from build123d import *

# Parameters (mm, degrees)
SKETCH_4_W               = 60
SKETCH_4_H               = 35
SKETCH_4_R               = 5
EXTRUDE_1_DEPTH          = 10
FILLET_1_R               = 10
FILLET_2_R               = 10
EXTRUDE_2_DEPTH          = 8
SKETCH_6_R               = 15
EXTRUDE_3_DEPTH          = 30
SKETCH_8_R               = 10
CUT_EXTRUDE_1_DEPTH      = 74.484692283
EXTRUDE_4_REACH          = 76.33
EXTRUDE_4_END_RADIUS     = 15
SKETCH_9_R               = 7.5
CUT_EXTRUDE_2_REACH      = 76.33
CUT_EXTRUDE_2_END_RADIUS = 10
SKETCH_10_R              = 5
RIB_START                = -2.5
RIB_1_DEPTH              = 5


# Read off the part's stored shape, not the designer's step: 筋1
with BuildPart() as part:
    # 草图4 → 凸台-拉伸1 (new body)
    with BuildSketch(Plane(origin=(0, 0, 0), x_dir=(1, 0, 0), z_dir=(0, 1, 0))):
        with Locations((0, 2.5)):
            Rectangle(SKETCH_4_W, SKETCH_4_H)
        with Locations(Location((-20, -5, 0), (0, 0, 270))):
            Circle(SKETCH_4_R, mode=Mode.SUBTRACT)
        with Locations(Location((20, -5, 0), (0, 0, 90))):
            Circle(SKETCH_4_R, mode=Mode.SUBTRACT)
    extrude(amount=EXTRUDE_1_DEPTH)

    # 圆角1
    fillet_1_edges = [part.edges().sort_by_distance(p)[0] for p in [
        (-30, 5, 15),
    ]]
    fillet(fillet_1_edges, radius=FILLET_1_R)

    # 圆角2
    fillet_2_edges = [part.edges().sort_by_distance(p)[0] for p in [
        (30, 5, 15),
    ]]
    fillet(fillet_2_edges, radius=FILLET_2_R)

    # 草图5 → 凸台-拉伸2 (add)
    with BuildSketch(Plane(origin=(0, 0, -20), x_dir=(-1, 0, 0), z_dir=(0, 0, -1))):
        with BuildLine():
            Line((-30, 10), (-13.945515037, 50.524727174))
            ThreePointArc((-13.945515037, 50.524727174), (0, 60), (13.945515037, 50.524727174))
            Line((13.945515037, 50.524727174), (30, 10))
            Line((30, 10), (-30, 10))
        make_face()
    extrude(amount=-EXTRUDE_2_DEPTH)

    # 草图6 → 凸台-拉伸3 (add)
    with BuildSketch(Plane(origin=(0, 0, -20), x_dir=(-1, 0, 0), z_dir=(0, 0, -1))):
        with Locations((0, 45)):
            Circle(SKETCH_6_R)
    extrude(amount=-EXTRUDE_3_DEPTH)

    # 草图8 → 切除-拉伸1 (cut, through all)
    with BuildSketch(Plane.XY.offset(10)):
        with Locations((0, 45)):
            Circle(SKETCH_8_R)
    extrude(amount=-CUT_EXTRUDE_1_DEPTH, mode=Mode.SUBTRACT)

    # 凸台-拉伸4: up to this cylinder (the profile starts outside it)
    extrude_4_end = Plane(origin=(0, 45, 0), z_dir=(0, 0, -1)) * Cylinder(EXTRUDE_4_END_RADIUS, 183.66, mode=Mode.PRIVATE)
    # 草图9 → 凸台-拉伸4 (add, up to the surface)
    with BuildSketch(Plane(origin=(0, 65, 0), x_dir=(1, 0, 0), z_dir=(0, 1, 0)), mode=Mode.PRIVATE) as extrude_4_sk1:
        with Locations(Location((0, 0, 0), (0, 0, 270))):
            Circle(SKETCH_9_R)
    extrude_4_tool1 = extrude(extrude_4_sk1.sketch, amount=-EXTRUDE_4_REACH, mode=Mode.PRIVATE) - extrude_4_end
    add(extrude_4_tool1.solids().sort_by_distance((0, 65, 0))[0])

    # 切除-拉伸2: up to this cylinder (the profile starts outside it)
    cut_extrude_2_end = Plane(origin=(0, 45, 0), z_dir=(0, 0, 1)) * Cylinder(CUT_EXTRUDE_2_END_RADIUS, 173.66, mode=Mode.PRIVATE)
    # 草图10 → 切除-拉伸2 (cut, up to the surface)
    with BuildSketch(Plane(origin=(0, 65, 0), x_dir=(1, 0, 0), z_dir=(0, 1, 0)), mode=Mode.PRIVATE) as cut_extrude_2_sk1:
        with Locations(Location((0, 0, 0), (0, 0, 270))):
            Circle(SKETCH_10_R)
    cut_extrude_2_tool1 = extrude(cut_extrude_2_sk1.sketch, amount=-CUT_EXTRUDE_2_REACH, mode=Mode.PRIVATE) - cut_extrude_2_end
    add(cut_extrude_2_tool1.solids().sort_by_distance((0, 65, 0))[0], mode=Mode.SUBTRACT)

    # 筋1 outline → 筋1 (add)
    with BuildSketch(Plane(origin=(0, 0, 0), x_dir=(0, 0, -1), z_dir=(1, 0, 0)).offset(RIB_START)):
        Polygon((-5, 32), (-5, 20), (-15, 10), (12, 10), (12, 32), align=None)
    extrude(amount=RIB_1_DEPTH)


solid = part.part
Build history of the part. All positions in model axes, mm. A direction names the side the tool comes from. Round coordinates to 2 decimals unless told otherwise and drop trailing zeros. Loops run counter-clockwise (first coordinate to the right, second up) from the corner with the lowest first, then second, coordinate; pieces in that order, holes last. Notation, with made-up numbers: (-33, 46) -> (-11, 46) arc R15 cw to (-11, 51) -> close; hole circle Ø7 at (-40, 40). An arc over 180 degrees is marked (long way). One line per item, written item: value. Start each with the question number.
Q1. Cut at B-B on y = 47. List the corners of the cut face in (x, z).
Q2. Drop flat-ended pins along their axis: pin 1 Ø3 at (y, z) = (49.5, -2.5) entering from +X; pin 2 Ø8 at (x, z) = (0, 0) entering from +Y; pin 3 Ø5 at (x, y) = (13, 34.5) entering from +Z. Give the stop position or say it passes through.
Q3. Cut at A-A on x = 0. List the corners of the cut face in (y, z).
Q4. Two-plate mould, pull along X, no slides. Class faces 5 (the face through (-5, 65, 2)), 6 (the face through (-21.86, 30.55, -16.06)), 7 (the face through (24.88, 4.93, 6.08)): released by +X, released by -X, zero draft, split by the parting line, or undercut.
Q5. Cut at C-C on z = 2. List the corners of the cut face in (x, y).
Q6. Cut at D-D on x = -22. List the corners of the cut face in (y, z), plus the area to 3 significant figures.
Q7. Probe line 1 along Z through (x, y) = (20, 5); line 2 along Z through (x, y) = (0, 62.25). List the from-to ranges inside material, lowest first.
Q8. 3-axis set-ups, long thin cutter, end or side, ignore diameter. For faces 1 (the face through (1.5, 59.41, 4.77)), 2 (the face through (2.5, 20, -1)), 3 (the face through (-16, 10, 1)), 4 (the face through (0, 15, 10)): which of +Z, -Z, +X, -X, +Y, -Y reach the whole face in a straight line?
Computed:
1. outline: (-15.34, -20) -> (-9.8, -20) -> (-9.8, 10) -> (-14.87, 10) -> (-14.87, -12) -> (-15.34, -12) -> close; (9.8, -20) -> (15.34, -20) -> (15.34, -12) -> (14.87, -12) -> (14.87, 10) -> (9.8, 10) -> close
2. pin 1: x = 14.7
2. pin 2: y = 35.83
2. pin 3: z = 10
3. outline: (0, -20) -> (35, -20) -> (35, 10) -> (30, 10) -> (30, 5) -> (20, 5) -> (10, 15) -> (0, 15) -> close; (55, -20) -> (60, -20) -> (60, -7.5) -> (65, -7.5) -> (65, -5) -> (55, -5) -> close; (55, 5) -> (65, 5) -> (65, 7.5) -> (60, 7.5) -> (60, 10) -> (55, 10) -> close
4. face 5: zero draft
4. face 6: released by -X
4. face 7: undercut
5. outline: (-30, 0) -> (-24, 0) -> (-24, 10) -> (-30, 10) -> close; (-16, 0) -> (16, 0) -> (16, 10) -> (2.5, 10) -> (2.5, 30.21) arc R15 ccw to (7.23, 58.14) -> (7.23, 65) -> (4.58, 65) -> (4.58, 53.89) arc R10 cw (long way) to (-4.58, 53.89) -> (-4.58, 65) -> (-7.23, 65) -> (-7.23, 58.14) arc R15 ccw to (-2.5, 30.21) -> (-2.5, 10) -> (-16, 10) -> close; (24, 0) -> (30, 0) -> (30, 10) -> (24, 10) -> close
6. outline: (0, -20) -> (30.19, -20) -> (30.19, -12) -> (10, -12) -> (10, 0.42) -> (0, 0.42) -> close; (0, 9.58) -> (10, 9.58) -> (10, 14.8) -> (0, 14.8) -> close
6. area: 418 mm²
7. line 1: -20 to 0, 10 to 15
7. line 2: -7.5 to -5, 5 to 7.5
8. face 1: +Y
8. face 2: +Z, +X
8. face 3: +Z, -X
8. face 4: +Z, +X, -X
